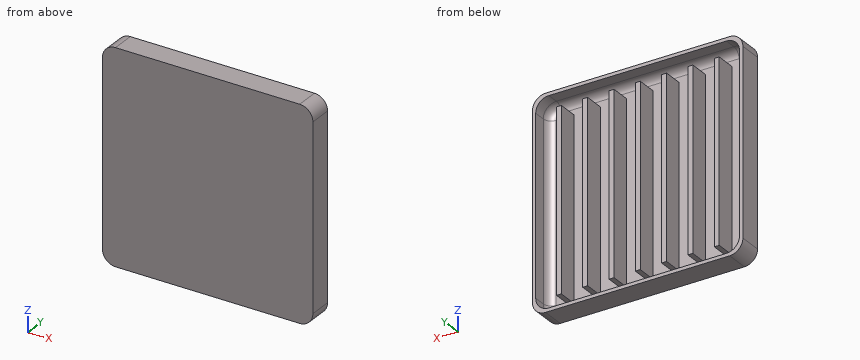
from build123d import *

# Parameters (mm, degrees)
ESQUISSE1_W                = 101.6
ESQUISSE1_H                = 101.6
BOSS_EXTRU_1_DEPTH         = 11.1125
CONG_1_R                   = 6.35
ENL_V_MAT_EXTRU_1_DEPTH    = 9.525
ESQUISSE4_W                = 2.38125
ESQUISSE4_H                = 87.3125
BOSS_EXTRU_3_DEPTH         = 9.525
R_P_TITION_LIN_AIRE1_COUNT = 7
R_P_TITION_LIN_AIRE1_PITCH = 12.7
CONG_2_R                   = 3.81


with BuildPart() as part:
    # Esquisse1 → Boss.-Extru.1 (new body)
    with BuildSketch(Plane(origin=(0, 0, 0), x_dir=(1, 0, 0), z_dir=(0, 1, 0))):
        Rectangle(ESQUISSE1_W, ESQUISSE1_H)
    extrude(amount=BOSS_EXTRU_1_DEPTH)

    # Congé1
    cong_1_edges = [part.edges().sort_by_distance(p)[0] for p in [
        (50.8, 5.55625, 50.8),
        (-50.8, 5.55625, 50.8),
        (-50.8, 5.55625, -50.8),
        (50.8, 5.55625, -50.8),
    ]]
    fillet(cong_1_edges, radius=CONG_1_R)

    # Esquisse2 → Enlèv. mat.-Extru.1 (cut)
    with BuildSketch(Plane(origin=(0, 11.1125, 0), x_dir=(1, 0, 0), z_dir=(0, 1, 0))):
        with BuildLine():
            Line((-42.8625, 49.2125), (42.8625, 49.2125))
            ThreePointArc((42.8625, 49.2125), (47.352628061, 47.352628061), (49.2125, 42.8625))
            Line((49.2125, 42.8625), (49.2125, -42.8625))
            ThreePointArc((49.2125, -42.8625), (47.352628061, -47.352628061), (42.8625, -49.2125))
            Line((42.8625, -49.2125), (-42.8625, -49.2125))
            ThreePointArc((-42.8625, -49.2125), (-47.352628061, -47.352628061), (-49.2125, -42.8625))
            Line((-49.2125, -42.8625), (-49.2125, 42.8625))
            ThreePointArc((-49.2125, 42.8625), (-47.352628061, 47.352628061), (-42.8625, 49.2125))
        make_face()
    extrude(amount=-ENL_V_MAT_EXTRU_1_DEPTH, mode=Mode.SUBTRACT)

    # Esquisse4 → Boss.-Extru.3 (add)
    with BuildSketch(Plane(origin=(0, 1.5875, 0), x_dir=(1, 0, 0), z_dir=(0, 1, 0))):
        with Locations((-38.179375, 0.79375)):
            Rectangle(ESQUISSE4_W, ESQUISSE4_H)
    boss_extru_3 = extrude(amount=BOSS_EXTRU_3_DEPTH)

    # Répétition linéaire1: Boss.-Extru.3 ×7
    with Locations(*[(i * R_P_TITION_LIN_AIRE1_PITCH, 0, 0) for i in range(1, R_P_TITION_LIN_AIRE1_COUNT)]):
        add(boss_extru_3)

    # Congé2
    cong_2_edges = [part.edges().sort_by_distance(p)[0] for p in [
        (-47.352628061, 1.5875, 47.352628061),
        (-49.2125, 1.5875, 0),
        (-47.352628061, 1.5875, -47.352628061),
        (0, 1.5875, -49.2125),
        (47.352628061, 1.5875, -47.352628061),
        (49.2125, 1.5875, 0),
        (47.352628061, 1.5875, 47.352628061),
        (0, 1.5875, 49.2125),
    ]]
    fillet(cong_2_edges, radius=CONG_2_R)


solid = part.part
CAD build for the part. Positions are in the model's coordinates, mm. Coordinates: 2 decimals unless noted, no trailing zeros. Write each loop counter-clockwise with the first axis right and the second up, starting at its lowest first coordinate (ties: lowest second). Pieces come first, ordered by that corner, then holes. Notation, with made-up numbers: M 40,55.5 L 48,55.5 A17 cw 48,68.5 Z; hole C 72.25,-14.75 d11. An arc over 180 degrees is marked long. Return JSON: item names as keys, results as strings.
Item 1: Slice it at A-A, the plane y = 8.25. State how many separate pieces and enclosed holes the cut face has, and give its area (3 significant figures).
Findings below:
{"separate pieces": "8", "enclosed holes": "1", "area": "2,090 mm2"}
Item 2: Probe line 1 (Z direction, x = -0.5, y = 6.5); line 2 (Z direction, x = 15, y = 8.5); line 3 (Y direction, x = -34, z = -23.5). List the from-to ranges inside material, lowest first. Write a range as from..to.
Findings below:
{"line 1": "z = -50.8..-49.21, -44.45..42.86, 49.21..50.8", "line 2": "z = -50.8..-49.21, 49.21..50.8", "line 3": "y = 0..1.59"}
Item 3: Slice it at B-B, the plane x = -17.5. Write the cut outline in (y, z).
Findings below:
{"outline": "M 0,-50.8 L 11.11,-50.8 L 11.11,-49.21 L 5.4,-49.21 A3.81 cw 1.59,-45.4 L 1.59,45.4 A3.81 cw 5.4,49.21 L 11.11,49.21 L 11.11,50.8 L 0,50.8 Z"}
Item 4: Drop a flat-ended pin along its axis: pin 1 Ø1 at (x, z) = (6.5, -38.5) entering from -Y. Give the stop position or say it passes through.
Findings below:
{"pin 1": "stops at y = 0"}
